from build123d import *


with BuildPart() as f1:
    # F0 (on Front) → F1 (revolve)
    with BuildSketch(Plane.XZ):
        with BuildLine():
            Line((0, 17.8337320685), (0, -54.8152588308))
            Line((0, -54.8152588308), (24.3101920933, -54.8152588308))
            Line((24.3101920933, -54.8152588308), (24.3101920933, -45.6168055534))
            Line((24.3101920933, -45.6168055534), (20.561552414, -45.6168055534))
            Line((20.561552414, -45.6168055534), (8.7669930706, -17.0896715711))
            Line((8.7669930706, -17.0896715711), (8.7669930706, -8.4479902372))
            ThreePointArc((8.7669930706, -8.4479902372), (11.4638422011, 4.0998815271), (1.4212700133, 12.0916788783))
            add(Edge.make_bspline(
                [(1.4212700133, 12.0916788783), (1.4424893444, 17.8337320685), (0, 17.8337320685)],
                knots=[4.6976782329, 4.6976782329, 4.6976782329, 6.2831853072, 6.2831853072, 6.2831853072], degree=2, weights=[1, 0.7018866658, 1]))
        make_face()
    revolve(axis=Axis((0, 0, 0.3754459321), (0, 0, -1)))


solid = f1.part
Source: CAD feature listing. Evaluate the final solid. Frame: model axes, mm. Round coordinates to 2 decimals unless told otherwise and drop trailing zeros. Loops run counter-clockwise (first coordinate to the right, second up) from the corner with the lowest first, then second, coordinate; pieces in that order, holes last. Notation, with made-up numbers: (75.5, 76) - (117.5, 76) arc R30 cw to (117.5, 113) - close; hole circle Ø1 at (78.25, 12.25). An arc over 180 degrees is marked (long way). Write item = value, one per line. Start each with the question number.
Item 1: First-contact query: pin 1 Ø8 at (x, z) = (4, -18.5) entering from -Y; pin 2 Ø5 at (y, z) = (8.5, -2) entering from -X; pin 3 Ø5 at (x, z) = (-14, -43.5) entering from -Y. Flat tips, straight axial feed; report the tip coordinate or a pass-through.
Item 2: Material intervals for line 1 (Z direction, x = 18.5, y = 15); line 2 (Z direction, x = -17.5, y = -8); line 3 (Y direction, x = -13.5, z = -51), sorted ascending.
Item 3: Mould query, pull axis Z, two halves, no side actions, for faces 1 (the face through (-1.9, 8.56, -12.71)), 2 (the face through (-19.292, 14.792, -50.152)), 3 (the face through (-20, -6, -45.617)), 4 (the face through (11.4, -3.6, -24.8)). Classes: released by +Z, released by -Z, zero draft, split by the parting line, or undercut.
Item 4: Section query A-A on z = -24.5. Output: boundary loops of the cut face in (x, y).
Results list:
q1.pin_1 = -10.6
q1.pin_2 = -10.46
q1.pin_3 = -20.75
q2.line_1 = -54.82 to -45.62
q2.line_2 = -54.82 to -42.42
q2.line_3 = -20.22 to 20.22
q3.face_1 = undercut
q3.face_2 = zero draft
q3.face_3 = released by +Z
q3.face_4 = undercut
q4.outline = circle Ø23.66 at (0, 0)
